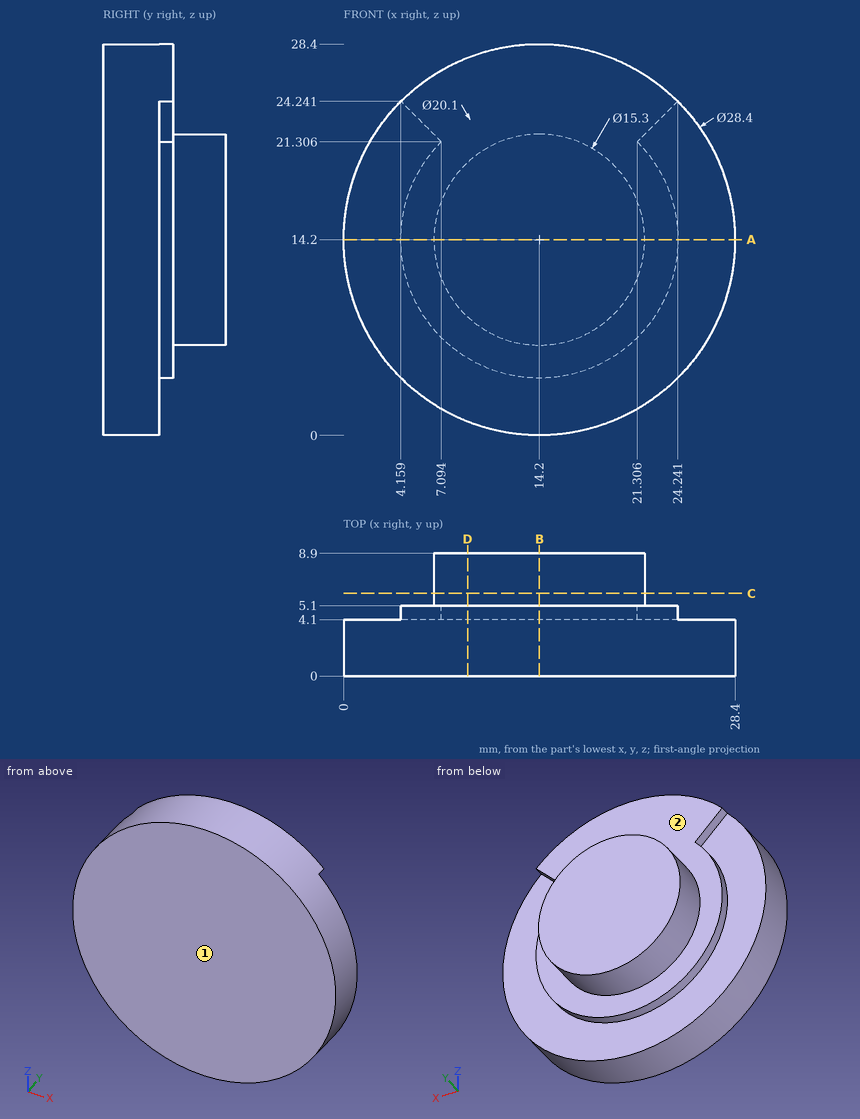
Here's the drawing with two shaded views (mm, measured from the low corner). I have some questions. A direction names the side the tool comes from. Give positions to 0.01 mm unless a question says otherwise; leave off trailing zeros. Write each loop counter-clockwise with the first axis right and the second up, starting at its lowest first coordinate (ties: lowest second). Pieces come first, ordered by that corner, then holes. Notation, with made-up numbers: (15.5, 56) -> (64.5, 56) arc R16 cw to (64.5, 67) -> close; hole circle Ø10 at (2, -30.75). An arc over 180 degrees is marked (long way). Answer as a JSON object with one key per item and string values. Group by question number.
Item 1: I'm going to push flat-ended pins straight in: P1, Ø1.5, axis at y = 2, z = 22, coming from the -X side; P2, Ø1.5, axis at x = 5.5, y = 3, coming from the -Z side (1 decimal); P3, Ø1.5, axis at x = 7.5, y = 7.5, coming from the +Z side. Where does each tip first touch, or does it pass through?
Item 2: Suppose I cut it at B-B (x = 14.2). Please give me the cut outline in (y, z), plus the area to 3 significant figures.
Item 3: Please list where these lines run through material, in increasing order: line 1 (Y direction, x = 10.75, z = 23.75); line 2 (Y direction, x = 24, z = 17); line 3 (X direction, y = 6.75, z = 7.25) (1 decimal). Write a range as [from, to].
Item 4: Suppose I cut it at A-A (z = 14.2). Please give me the cut outline in (x, y).
Item 5: Suppose I cut it at D-D (x = 9). Please give me the cut outline in (y, z), plus the area to 3 significant figures.
Item 6: For the marked faces 1 and 2, which set-ups out of +Z, -Z, +X, -X, +Y, -Y let a thin tool reach every point of the face, with its end or its side?
Item 7: Suppose I cut it at C-C (y = 6). Please give me the cut outline in (x, z).
Findings:
{
 "1": {"P1": "stops at x = 1.87", "P2": "stops at z = 2.4", "P3": "stops at z = 19.01"},
 "2": {"outline": "(0, 0) -> (4.1, 0) -> (4.1, 4.15) -> (5.1, 4.15) -> (5.1, 6.55) -> (8.9, 6.55) -> (8.9, 21.85) -> (5.1, 21.85) -> (5.1, 28.4) -> (0, 28.4) -> close", "area": "199 mm²"},
 "3": {"line 1": "y = [0, 5.1]", "line 2": "y = [0, 4.1]", "line 3": "x = [11, 17.4]"},
 "4": {"outline": "(0, 0) -> (28.4, 0) -> (28.4, 4.1) -> (24.25, 4.1) -> (24.25, 5.1) -> (21.85, 5.1) -> (21.85, 8.9) -> (6.55, 8.9) -> (6.55, 5.1) -> (4.15, 5.1) -> (4.15, 4.1) -> (0, 4.1) -> close"},
 "5": {"outline": "(0, 0.99) -> (4.1, 0.99) -> (4.1, 5.6) -> (5.1, 5.6) -> (5.1, 8.59) -> (8.9, 8.59) -> (8.9, 19.81) -> (5.1, 19.81) -> (5.1, 27.41) -> (0, 27.41) -> close", "area": "173 mm²"},
 "6": {"face 1": "+Z, -Z, +X, -X, -Y", "face 2": "+Y"},
 "7": {"outline": "circle Ø15.3 at (14.2, 14.2)"}
}
